Part model, mm, in its own coordinate system. A direction names the side the tool comes from. Coordinates: 2 decimals unless noted, no trailing zeros. Loops run counter-clockwise (first coordinate to the right, second up) from the corner with the lowest first, then second, coordinate; pieces in that order, holes last. Notation, with made-up numbers: (3, 10) -> (23, 10) arc R25 ccw to (23, 28) -> close; hole circle Ø4 at (72.25, -7). An arc over 180 degrees is marked (long way). One line per question, with ' | ' between items. Start each with the question number.
1) 3-axis set-ups, long thin cutter, end or side, ignore diameter. For faces 4 (the face through (15, 16, 0)), 5 (the face through (22, 17, 0)), 6 (the face through (9, 0, 0)): which of +Z, -Z, +X, -X, +Y, -Y reach the whole face in a straight line?
2) Cut at B-B (x = 28). List the corners of the cut face in (y, z).
3) Two-plate mould, pull along Z, no slides. Class faces 1 (the face through (25, 21, 1)), 2 (the face through (17.5, -20, 2.9)), 3 (the face through (34.99, 20.94, 0.77)): released by +Z, released by -Z, zero draft, split by the parting line, or undercut.
4) Cut at D-D (y = 11.5). List the corners of the cut face in (x, z).
5) Probe L1, parallel to X at y = 22, z = 0; L2, parallel to Y at x = 8, z = -25; L3, parallel to Z at x = 13, y = -17.5. List the from-to ranges inside material, lowest first. Write a range as from..to.
6) Cut at A-A (z = 0). List the corners of the cut face in (x, y).
7) Drop flat-ended pins along their axis: pin 1 (1.5 mm diameter, centred on y = 18, z = 15, fed in from +X); pin 2 (6 mm diameter, centred on x = 18, y = -7, fed in from -Z); pin 3 (5 mm diameter, centred on x = 7, z = 0.5, fed in from -Y); pin 4 (5.5 mm diameter, centred on x = 28, z = 0, fed in from +Y). Give the stop position or say it passes through.
8) Cut at C-C (x = 10.5). List the corners of the cut face in (y, z).
from build123d import *

# Parameters (mm, degrees)
BASE_R_VOLUTION_ANGLE   = 180
ESQUISSE2_R             = 3.16227766
ENL_V_MAT_EXTRU_1_DEPTH = 67.895440801


with BuildPart() as part:
    # Esquisse1 → Base-Révolution (revolve)
    with BuildSketch(Plane(origin=(0, 0, 0), x_dir=(0, 0, -1), z_dir=(1, 0, 0))):
        Polygon((-7, 0), (-7, 6), (-15, 6), (-15, 25), (-35, 25), (-35, 17), (-20, 17), (-20, -20), (-17.5, -20), (-17.5, 0), align=None)
    revolve(axis=Axis((0, 0, 0), (0, 1, 0)), revolution_arc=BASE_R_VOLUTION_ANGLE)

    # Esquisse2 → Enlèv. mat.-Extru.1 (cut, through all)
    with BuildSketch(Plane(origin=(0, 25, 0), x_dir=(-1, 0, 0), z_dir=(0, 1, 0))):
        with Locations((0, -28)):
            Circle(ESQUISSE2_R)
        with Locations((0, 28)):
            Circle(ESQUISSE2_R)
        with Locations(Location((-28, 0, 0), (0, 0, 90))):
            Circle(ESQUISSE2_R)
    extrude(amount=-ENL_V_MAT_EXTRU_1_DEPTH, mode=Mode.SUBTRACT)


solid = part.part
Reported:
1) face 4: -X, +Y | face 5: +X, -Y | face 6: -X, -Y
2) outline: (17, -21) -> (25, -21) -> (25, -3.16) -> (17, -3.16) -> close; (17, 3.16) -> (25, 3.16) -> (25, 21) -> (17, 21) -> close
3) face 1: undercut | face 2: zero draft | face 3: split by the parting line
4) outline: (0, -20) arc R20 ccw to (0, 20) -> (0, 15) arc R15 cw to (0, -15) -> close
5) L1: x = 15..24.84, 31.16..35 | L2: y = 17..25 | L3: z = -15.2..-11.72, 11.72..15.2
6) outline: (7, 0) -> (17.5, 0) -> (17.5, -20) -> (20, -20) -> (20, 17) -> (24.84, 17) -> (24.84, 25) -> (15, 25) -> (15, 6) -> (7, 6) -> close; (31.16, 17) -> (35, 17) -> (35, 25) -> (31.16, 25) -> close
7) pin 1: stops at x = 31.97 | pin 2: stops at z = -13.23 | pin 3: stops at y = 0 | pin 4: passes through
8) outline: (-20, -17.02) -> (17, -17.02) -> (17, -33.39) -> (25, -33.39) -> (25, -10.71) -> (6, -10.71) -> (6, 10.71) -> (25, 10.71) -> (25, 33.39) -> (17, 33.39) -> (17, 17.02) -> (-20, 17.02) -> (-20, 14) -> (0, 14) -> (0, -14) -> (-20, -14) -> close
